```python
from build123d import *

# Parameters (mm, degrees)
CROQUIS7_W              = 92
CROQUIS7_H              = 48
CROQUIS7_W_2            = 74
CROQUIS7_H_2            = 29
SALIENTE_EXTRUIR5_DEPTH = 25
CROQUIS8_W              = 82
CROQUIS8_H              = 38
CORTAR_EXTRUIR3_DEPTH   = 18
REDONDEO1_R             = 5
REDONDEO2_R             = 1
CROQUIS10_W             = 10
CROQUIS10_H             = 10
CORTAR_EXTRUIR4_DEPTH   = 20


with BuildPart() as part:
    # Croquis7 → Saliente-Extruir5 (new body)
    with BuildSketch(Plane.XY):
        with Locations((37, -13)):
            Rectangle(CROQUIS7_W, CROQUIS7_H)
        with Locations((37, -14.5)):
            Rectangle(CROQUIS7_W_2, CROQUIS7_H_2, mode=Mode.SUBTRACT)
    extrude(amount=SALIENTE_EXTRUIR5_DEPTH)

    # Croquis8 → Cortar-Extruir3 (cut)
    with BuildSketch(Plane.XY.offset(25)):
        with Locations((37, -13)):
            Rectangle(CROQUIS8_W, CROQUIS8_H)
    extrude(amount=-CORTAR_EXTRUIR3_DEPTH, mode=Mode.SUBTRACT)

    # Redondeo1
    redondeo1_edges = [part.edges().sort_by_distance(p)[0] for p in [
        (-9, 11, 12.5),
        (83, 11, 12.5),
        (83, -37, 12.5),
        (-9, -37, 12.5),
    ]]
    fillet(redondeo1_edges, radius=REDONDEO1_R)

    # Redondeo2
    redondeo2_edges = [part.edges().sort_by_distance(p)[0] for p in [
        (-4, -32, 16),
        (-4, 6, 16),
        (78, 6, 16),
        (78, -32, 16),
    ]]
    fillet(redondeo2_edges, radius=REDONDEO2_R)

    # Croquis10 → Cortar-Extruir4 (cut)
    with BuildSketch(Plane(origin=(83, 0, 0), x_dir=(0, 0, -1), z_dir=(1, 0, 0))):
        with Locations((-25, -13)):
            Rectangle(CROQUIS10_W, CROQUIS10_H)
    extrude(amount=-CORTAR_EXTRUIR4_DEPTH, mode=Mode.SUBTRACT)


solid = part.part
```
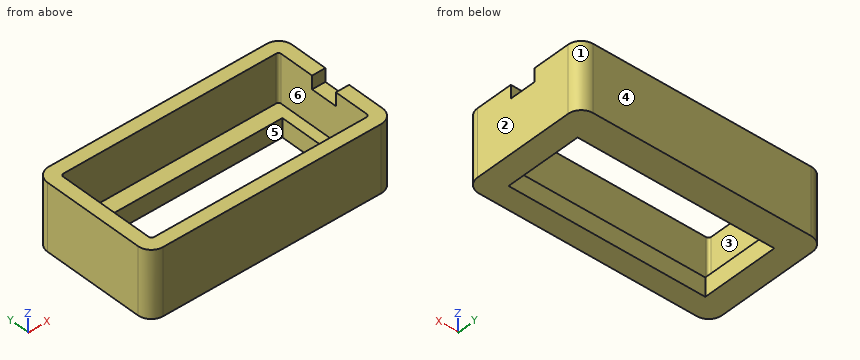
The model under review builds one solid part; all positions refer to its coordinate system, in mm. Face numbers are marked on the shaded views. A direction names the side the tool comes from. Coordinates: 2 decimals unless noted, no trailing zeros. Write each loop counter-clockwise with the first axis right and the second up, starting at its lowest first coordinate (ties: lowest second). Pieces come first, ordered by that corner, then holes.
1) Clearance check with flat-ended pins moving along their axes: pin 1 Ø1.5 at (x, z) = (81, 21.5) entering from +Y; pin 2 Ø1.5 at (x, y) = (80, -14) entering from +Z. State where each tip first meets the part, or that it passes through.
2) We need section D-D on y = 2. State the section outline as (x, z) points.
3) Machinability: for the marked faces 4, 5 and 6, which of the approach directions +Z, -Z, +X, -X, +Y, -Y give a long, thin tool a straight path to every point of the face, cutting with its end or side? Answer none if there is none.
4) The part is to be moulded in two halves that separate along Y. For the marked faces 1, 2 and 3, say which applies: pulls with the +Y half, pulls with the -Y half, needs draft (parallel to the pull), parting line crosses it, or undercut.
5) To check wall thickness, follow probe 1 along X at (y, z) = (3, 16); probe 2 along X at (y, z) = (-13, 6); probe 3 along Y at (x, z) = (0.5, 13). State the ranges of each line that lie inside material, in increasing order.
6) We need section A-A on y = -14. State the section outline as (x, z) points.
7) We need section C-C on x = 34.5. State the section outline as (y, z) points, then the cut area to 3 significant figures.
8) We need section B-B on z = 19. State the section outline as (x, y) points.
Answer list:
1. pin 1: stops at y = 10.47
1. pin 2: stops at z = 20
2. outline: (-9, 0) - (83, 0) - (83, 25) - (78, 25) - (78, 7) - (-4, 7) - (-4, 25) - (-9, 25) - close
3. face 4: +Z, -Z, +X, -X, +Y
3. face 5: +Z, -Z
3. face 6: +Z
4. face 1: pulls with the +Y half
4. face 2: needs draft
4. face 3: undercut
5. probe 1: x = -9 to -4, 78 to 83
5. probe 2: x = -9 to 0, 74 to 83
5. probe 3: y = -37 to -32, 6 to 11
6. outline: (-9, 0) - (0, 0) - (0, 7) - (-4, 7) - (-4, 25) - (-9, 25) - close; (74, 0) - (83, 0) - (83, 20) - (78, 20) - (78, 7) - (74, 7) - close
7. outline: (-37, 0) - (-29, 0) - (-29, 7) - (-32, 7) - (-32, 25) - (-37, 25) - close; (0, 0) - (11, 0) - (11, 25) - (6, 25) - (6, 7) - (0, 7) - close
7. area: 313 mm2
8. outline: (-9, -32) arc R5 ccw to (-4, -37) - (78, -37) arc R5 ccw to (83, -32) - (83, 6) arc R5 ccw to (78, 11) - (-4, 11) arc R5 ccw to (-9, 6) - close; hole (-4, -31) arc R1 ccw to (-3, -32) - (77, -32) arc R1 ccw to (78, -31) - (78, 5) arc R1 ccw to (77, 6) - (-3, 6) arc R1 ccw to (-4, 5) - close
